Source: CAD feature listing. Evaluate the final solid. Frame: model axes, mm. Coordinates: 2 decimals unless noted, no trailing zeros. Write each loop counter-clockwise with the first axis right and the second up, starting at its lowest first coordinate (ties: lowest second). Pieces come first, ordered by that corner, then holes. Notation, with made-up numbers: (87, 41) -> (144, 41) arc R19 cw to (144, 78) -> close; hole circle Ø2 at (21.25, -12). An arc over 180 degrees is marked (long way). One line per item, written item: value. Start each with the question number.
1. Section query B-B, the plane y = 0.95. Output: boundary loops of the cut face in (x, z).
2. Line query: line 1 (X direction, y = 1.05, z = 0.5); line 2 (X direction, y = 2, z = 2); line 3 (Z direction, x = -10, y = -0.95). Output: solid intervals per line, ascending.
3. Section query A-A, the plane z = 0. Output: boundary loops of the cut face in (x, y), and give its area (3 significant figures).
4. Section query C-C, the plane x = -10. Output: boundary loops of the cut face in (y, z).
5. First-contact query: P1, Ø7, axis at x = -10, z = 0, coming from the +Y side; P2, Ø2, axis at x = -46.5, y = 1.5, coming from the -Z side. Flat tips, straight axial feed; report the tip coordinate or a pass-through.
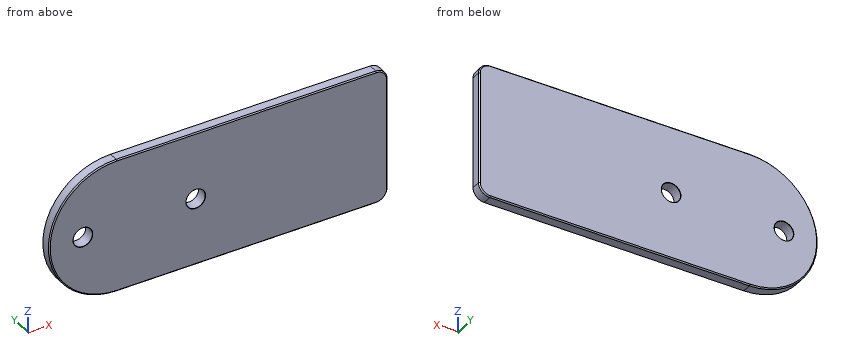
from build123d import *

# Parameters (mm, degrees)
F0_R     = 4.25
F1_DEPTH = 2.5
F2_R     = 5
F3_SIZE  = 0.5
F4_SIZE  = 0.1


with BuildPart() as f1:
    # F0 (on Front) → F1 (new body, symmetric)
    with BuildSketch(Plane.XZ):
        with BuildLine():
            Line((75, -30), (75, 30))
            Line((75, 30), (-45, 30))
            ThreePointArc((-45, 30), (-75, 0), (-45, -30))
            Line((-45, -30), (75, -30))
        make_face()
        with Locations((-60, 0)):
            Circle(F0_R, mode=Mode.SUBTRACT)
        with Locations((-10, 0)):
            Circle(F0_R, mode=Mode.SUBTRACT)
    extrude(amount=F1_DEPTH, both=True)

    # F2
    f2_edges = [f1.edges().sort_by_distance(p)[0] for p in [
        (75, 0, -30),
        (75, 0, 30),
    ]]
    fillet(f2_edges, radius=F2_R)

    # F3
    f3_edges = [f1.edges().sort_by_distance(p)[0] for p in [
        (12.5, -2.5, -30),
        (12.5, 2.5, 30),
    ]]
    chamfer(f3_edges, length=F3_SIZE)

    # F4
    f4_edges = [f1.edges().sort_by_distance(p)[0] for p in [
        (-14.25, 2.5, 0),
        (-64.25, 2.5, 0),
        (-64.25, -2.5, 0),
        (-14.25, -2.5, 0),
    ]]
    chamfer(f4_edges, length=F4_SIZE)


solid = f1.part
Computed values:
1. outline: (-45, -30) -> (70, -30) arc R5 ccw to (75, -25) -> (75, 25) arc R5 ccw to (70, 30) -> (-45, 30) arc R30 ccw to start; hole circle Ø8.5 at (-60, 0); hole circle Ø8.5 at (-10, 0)
2. line 1: x = -75 to -64.22, -55.78 to -14.22, -5.78 to 75
2. line 2: x = -74.93 to -63.75, -56.25 to -13.75, -6.25 to 75
2. line 3: z = -30 to -4.25, 4.25 to 30
3. outline: (-75, -2) -> (-74.5, -2.5) -> (-64.35, -2.5) -> (-64.25, -2.4) -> (-64.25, 2.4) -> (-64.35, 2.5) -> (-74.5, 2.5) -> (-75, 2) -> close; (-55.75, -2.4) -> (-55.65, -2.5) -> (-14.35, -2.5) -> (-14.25, -2.4) -> (-14.25, 2.4) -> (-14.35, 2.5) -> (-55.65, 2.5) -> (-55.75, 2.4) -> close; (-5.75, -2.4) -> (-5.65, -2.5) -> (74.5, -2.5) -> (75, -2) -> (75, 2) -> (74.5, 2.5) -> (-5.65, 2.5) -> (-5.75, 2.4) -> close
3. area: 664 mm²
4. outline: (-2.5, -29.5) -> (-2, -30) -> (2, -30) -> (2.5, -29.5) -> (2.5, -4.35) -> (2.4, -4.25) -> (-2.4, -4.25) -> (-2.5, -4.35) -> close; (-2.5, 4.35) -> (-2.4, 4.25) -> (2.4, 4.25) -> (2.5, 4.35) -> (2.5, 29.5) -> (2, 30) -> (-2, 30) -> (-2.5, 29.5) -> close
5. P1: passes through
5. P2: stops at z = -30
